For this review, take the finished solid that the model builds, in its own axes (mm). A direction names the side the tool comes from. Give positions to 0.01 mm unless a question says otherwise; leave off trailing zeros. Write each loop counter-clockwise with the first axis right and the second up, starting at its lowest first coordinate (ties: lowest second). Pieces come first, ordered by that corner, then holes.
1) Machinability: for faces 4 (the face through (2, -8, 43.74)), 5 (the face through (64.77, -8, 51)), 6 (the face through (47, -8, 1.524)), 7 (the face through (0, -2, 26)), 8 (the face through (47, -8, 3.556)), which of the approach directions +Z, -Z, +X, -X, +Y, -Y give a long, thin tool a straight path to every point of the face, cutting with its end or side? Answer none if there is none.
2) We need section A-A on x = 66.04. Give the boundary of the cut face in (y, z).
3) Wall thickness on line 1 along Z through (x, y) = (66.04, -1.4); line 2 along Z through (x, y) = (40.5, -8.75); line 3 along Z through (x, y) = (13.97, -1.75): over which ranges is each line inside the solid? List them lowest first.
4) We need section D-D on z = 7.62. Give the boundary of the cut face in (x, y), and give its area (3 significant figures).
5) For P1, Ø0.6, axis at y = -8.5, z = 51, coming from the +X side; P2, Ø7, axis at x = 38.5, y = -9, coming from the +Z side; P3, Ø2, axis at x = 3.5, y = -6, coming from the +Z side, all flat-tipped, find the tip position at first contact; note any pin that passes through.
6) We need section B-B on y = -4.5. Give the boundary of the cut face in (x, z).
7) We need section C-C on z = 50.8. Give the boundary of the cut face in (x, y), and give its area (3 significant figures).
8) Draft analysis for pull direction Z (two halves, no side actions). For faces 1 (the face through (15.436, -1.528, 1.932)), 2 (the face through (34, -2, 53.34)), 3 (the face through (42, -12.1, 51)), state which applies: pulls with the +Z half, pulls with the -Z half, needs draft (parallel to the pull), parting line crosses it, or undercut.
from build123d import *

# Parameters (mm, degrees)
F0_W     = 68.58
F0_H     = 53.34
F0_R     = 1.5875
F1_DEPTH = 3.1
F2_W     = 6.2
F2_H     = 12
F2_W_2   = 9.8
F2_W_3   = 11.2
F2_H_2   = 8.9
F2_W_4   = 1.8
F3_DEPTH = 10.9
F4_W     = 44.704
F4_H     = 2.032
F4_W_2   = 35.56
F5_DEPTH = 9


with BuildPart() as f1:
    # F0 (on Front) → F1 (new body)
    with BuildSketch(Plane.XZ):
        with Locations((34.29, 26.67)):
            Rectangle(F0_W, F0_H)
        with Locations((13.97, 2.54)):
            Circle(F0_R, mode=Mode.SUBTRACT)
        with Locations((66.04, 7.62)):
            Circle(F0_R, mode=Mode.SUBTRACT)
        with Locations((15.24, 50.8)):
            Circle(F0_R, mode=Mode.SUBTRACT)
        with Locations((66.04, 35.56)):
            Circle(F0_R, mode=Mode.SUBTRACT)
    extrude(amount=F1_DEPTH)

    # F2 (on face) → F3 (join)
    with BuildSketch(Plane.XZ.offset(3.1)):
        with Locations((-3.1, 37.74)):
            Rectangle(F2_W, F2_H)
        with Locations((4.9, 37.74)):
            Rectangle(F2_W_2, F2_H)
        with Locations((5.6, 7.75)):
            Rectangle(F2_W_3, F2_H_2)
        with Locations((-0.9, 7.75)):
            Rectangle(F2_W_4, F2_H_2)
    extrude(amount=F3_DEPTH)

    # F4 (on face) → F5 (join)
    with BuildSketch(Plane.XZ.offset(3.1)):
        with Locations((42.418, 50.8)):
            Rectangle(F4_W, F4_H)
        with Locations((46.99, 2.54)):
            Rectangle(F4_W_2, F4_H)
    extrude(amount=F5_DEPTH)


solid = f1.part
Results list:
1. face 4: +Z, +X, -X, -Y
1. face 5: +Z, -Z, +X, -Y
1. face 6: -Z, +X, -X, -Y
1. face 7: +Z, -Z, -X, +Y
1. face 8: +X, -Y
2. outline: (-3.1, 0) - (0, 0) - (0, 6.03) - (-3.1, 6.03) - close; (-3.1, 9.21) - (0, 9.21) - (0, 33.97) - (-3.1, 33.97) - close; (-3.1, 37.15) - (0, 37.15) - (0, 53.34) - (-3.1, 53.34) - close
3. line 1: z = 0 to 6.03, 9.21 to 33.97, 37.15 to 53.34
3. line 2: z = 1.52 to 3.56, 49.78 to 51.82
3. line 3: z = 0 to 0.95, 4.13 to 49.85, 51.75 to 53.34
4. outline: (-1.8, -14) - (11.2, -14) - (11.2, -3.1) - (64.45, -3.1) - (64.45, 0) - (0, 0) - (0, -3.1) - (-1.8, -3.1) - close; (67.63, -3.1) - (68.58, -3.1) - (68.58, 0) - (67.63, 0) - close
4. area: 344 mm2
5. P1: stops at x = 64.77
5. P2: stops at z = 51.82
5. P3: stops at z = 43.74
6. outline: (-6.2, 31.74) - (9.8, 31.74) - (9.8, 43.74) - (-6.2, 43.74) - close; (-1.8, 3.3) - (11.2, 3.3) - (11.2, 12.2) - (-1.8, 12.2) - close; (20.07, 49.78) - (64.77, 49.78) - (64.77, 51.82) - (20.07, 51.82) - close; (29.21, 1.52) - (64.77, 1.52) - (64.77, 3.56) - (29.21, 3.56) - close
7. outline: (0, -3.1) - (13.65, -3.1) - (13.65, 0) - (0, 0) - close; (16.83, -3.1) - (20.07, -3.1) - (20.07, -12.1) - (64.77, -12.1) - (64.77, -3.1) - (68.58, -3.1) - (68.58, 0) - (16.83, 0) - close
7. area: 605 mm2
8. face 1: undercut
8. face 2: pulls with the +Z half
8. face 3: needs draft
